```python
from build123d import *

# Parameters (mm, degrees)
F0_W     = 286
F0_H     = 180
F1_DEPTH = 6.2
F2_W     = 12
F2_H     = 6.2
F2_W_2   = 5
F3_DEPTH = 6.201
F4_W     = 12
F4_H     = 6.2
F5_DEPTH = 6.2
F6_W     = 6.2
F6_H     = 12
F7_DEPTH = 6.2


with BuildPart() as f1:
    # F0 (on Front) → F1 (new body)
    with BuildSketch(Plane.XZ):
        Rectangle(F0_W, F0_H)
    extrude(amount=F1_DEPTH)

    # F2 (on face) → F3 (cut, through all)
    with BuildSketch(Plane.XZ.offset(6.2)):
        with Locations((-120, -25.4)):
            Rectangle(F2_W, F2_H)
        with Locations((-96, -25.4)):
            Rectangle(F2_W, F2_H)
        with Locations((-72, -25.4)):
            Rectangle(F2_W, F2_H)
        with Locations((-48, -25.4)):
            Rectangle(F2_W, F2_H)
        with Locations((-24, -25.4)):
            Rectangle(F2_W, F2_H)
        with Locations((0, -25.4)):
            Rectangle(F2_W, F2_H)
        with Locations((24, -25.4)):
            Rectangle(F2_W, F2_H)
        with Locations((48, -25.4)):
            Rectangle(F2_W, F2_H)
        with Locations((72, -25.4)):
            Rectangle(F2_W, F2_H)
        with Locations((96, -25.4)):
            Rectangle(F2_W, F2_H)
        with Locations((120, -25.4)):
            Rectangle(F2_W, F2_H)
        with Locations((-140.5, -25.4)):
            Rectangle(F2_W_2, F2_H)
        with Locations((140.5, -25.4)):
            Rectangle(F2_W_2, F2_H)
    extrude(amount=-F3_DEPTH, mode=Mode.SUBTRACT)

    # F4 (on face) → F5 (join, through all)
    with BuildSketch(Plane.XZ.offset(6.2)):
        with Locations((-132, -93.1)):
            Rectangle(F4_W, F4_H)
        with Locations((-108, -93.1)):
            Rectangle(F4_W, F4_H)
        with Locations((-84, -93.1)):
            Rectangle(F4_W, F4_H)
        with Locations((-60, -93.1)):
            Rectangle(F4_W, F4_H)
        with Locations((-36, -93.1)):
            Rectangle(F4_W, F4_H)
        with Locations((-12, -93.1)):
            Rectangle(F4_W, F4_H)
        with Locations((12, -93.1)):
            Rectangle(F4_W, F4_H)
        with Locations((36, -93.1)):
            Rectangle(F4_W, F4_H)
        with Locations((60, -93.1)):
            Rectangle(F4_W, F4_H)
        with Locations((84, -93.1)):
            Rectangle(F4_W, F4_H)
        with Locations((108, -93.1)):
            Rectangle(F4_W, F4_H)
        with Locations((132, -93.1)):
            Rectangle(F4_W, F4_H)
    extrude(amount=-F5_DEPTH)

    # F6 (on face) → F7 (join)
    with BuildSketch(Plane.XZ.offset(6.2)):
        with Locations((-146.1, 0)):
            Rectangle(F6_W, F6_H)
        with Locations((-146.1, 24)):
            Rectangle(F6_W, F6_H)
        with Locations((-146.1, 48)):
            Rectangle(F6_W, F6_H)
        with Locations((-146.1, 72)):
            Rectangle(F6_W, F6_H)
        with Locations((-146.1, -24)):
            Rectangle(F6_W, F6_H)
        with Locations((-146.1, -48)):
            Rectangle(F6_W, F6_H)
        with Locations((-146.1, -72)):
            Rectangle(F6_W, F6_H)
        with Locations((146.1, 0)):
            Rectangle(F6_W, F6_H)
        with Locations((146.1, 24)):
            Rectangle(F6_W, F6_H)
        with Locations((146.1, -24)):
            Rectangle(F6_W, F6_H)
        with Locations((146.1, -72)):
            Rectangle(F6_W, F6_H)
        with Locations((146.1, -48)):
            Rectangle(F6_W, F6_H)
        with Locations((146.1, 72)):
            Rectangle(F6_W, F6_H)
        with Locations((146.1, 48)):
            Rectangle(F6_W, F6_H)
    extrude(amount=-F7_DEPTH)


solid = f1.part
```
Read the model definition and answer for the solid it produces. Units are mm, in the model's axes. A direction names the side the tool comes from. Give positions to 0.01 mm unless a question says otherwise; leave off trailing zeros. Write each loop counter-clockwise with the first axis right and the second up, starting at its lowest first coordinate (ties: lowest second). Pieces come first, ordered by that corner, then holes. Notation, with made-up numbers: M 44,78.5 L 78,78.5 A14 cw 78,101.5 Z; hole C 85.25,22.25 d4. An arc over 180 degrees is marked long. Put each result on its own line as item: value. Start each with the question number.
1. The part is cut by section C-C, the plane z = -10.5. Give the vertices of the cut face in (x, y).
2. Which of the six approach directions +Z, -Z, +X, -X, +Y, -Y give full straight-line access (tool end or side, diameter ignored) to faces 1 (the flat face through (96, -3, -28.5)), 2 (the flat face through (72, -3, -90)), 3 (the flat face through (146, -3, 30))?
3. The part is cut by section B-B, the plane y = -3.5. Give the number of separate pieces and of enclosed holes in the cut face, and give its area (3 significant figures).
4. The part is cut by section A-A, the plane x = -2. Give the vertices of the cut face in (y, z), and give its area (3 significant figures).
5. For a pull along Z with two mould halves and no side action, classify faces 4 (the flat face through (-126, -3, -25)), 5 (the flat face through (-24, -3, -28.5)), 6 (the flat face through (-6, -3, -93)), 7 (the flat face through (-96, -3, -90)) as released by +Z, released by -Z, zero draft, split by the parting line, or undercut.
6. Each of these flat-tipped pins is pushed along its axis until it touches: pin 1 Ø1.9 at (y, z) = (-2.5, -33) entering from +X; pin 2 Ø3 at (x, y) = (-145.5, -2) entering from +Z; pin 3 Ø3 at (y, z) = (-4, -93) entering from +X. Where does it stop, or does it pass through?
7. Consider line 1 along Z through (x, y) = (-95, -2); line 2 along X through (y, z) = (-4.5, -35). Determine where each line is inside the solid, lowest interval first.
Final values:
1. outline: M -143,-6.2 L 143,-6.2 L 143,0 L -143,0 Z
2. face 1: +Y, -Y
2. face 2: -Z, +Y, -Y
2. face 3: +X, +Y, -Y
3. separate pieces: 1
3. enclosed holes: 13
3. area: 52,500 mm²
4. outline: M -6.2,-90 L 0,-90 L 0,-28.5 L -6.2,-28.5 Z; M -6.2,-22.3 L 0,-22.3 L 0,90 L -6.2,90 Z
4. area: 1,080 mm²
5. face 4: undercut
5. face 5: undercut
5. face 6: zero draft
5. face 7: released by -Z
6. pin 1: stops at x = 143
6. pin 2: stops at z = 78
6. pin 3: stops at x = 138
7. line 1: z = -90 to -28.5, -22.3 to 90
7. line 2: x = -143 to 143
